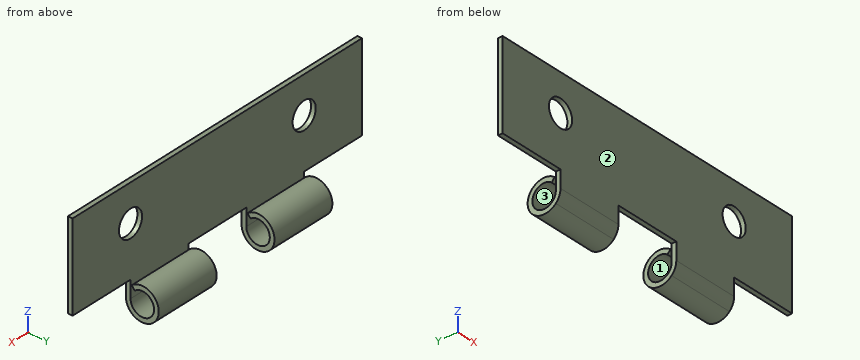
```python
from build123d import *

# Parameters (mm, degrees)
SKETCH_1_R             = 2
SM_BASE_FLANGE_1_DEPTH = 0.7
OTHER_START            = -15
OTHER_2_DEPTH          = 30
OTHER_2_2_DEPTH        = 10
OTHER_START_2          = 5
OTHER_2_3_DEPTH        = 10


# Read off the part's stored shape, not the designer's step: 褶边2
# Sheet-metal steps are written as plain solids
with BuildPart() as part:
    # Sketch 1 → 基体-法兰1 (new body)
    with BuildSketch(Plane(origin=(0, 0, 0), x_dir=(1, 0, 0), z_dir=(0, 1, 0))):
        Polygon((-25, 0), (25, 0), (25, 13), (15, 13), (15, 18), (5, 18), (5, 13), (-5, 13), (-5, 18), (-15, 18), (-15, 13), (-25, 13), align=None)
        with Locations(Location((-15, 5.5, 0), (0, 0, 270))):
            Circle(SKETCH_1_R, mode=Mode.SUBTRACT)
        with Locations(Location((15, 5.5, 0), (0, 0, 90))):
            Circle(SKETCH_1_R, mode=Mode.SUBTRACT)
    extrude(amount=-SM_BASE_FLANGE_1_DEPTH)

    # Other 2 outline → Other 2 (cut)
    with BuildSketch(Plane.YZ.offset(OTHER_START)):
        with BuildLine():
            Line((0, -18), (0, -17.264642819))
            ThreePointArc((0, -17.264642819), (-0.518259244, -16.476012959), (-0.7, -15.55))
            Line((-0.7, -15.55), (-0.7, -18))
            Line((-0.7, -18), (0, -18))
        make_face()
    extrude(amount=OTHER_2_DEPTH, mode=Mode.SUBTRACT)

    # Other 2 2 outline → Other 2 2 (add)
    with BuildSketch(Plane.YZ.offset(OTHER_START)):
        with BuildLine():
            Line((0.175170356, -13.673191114), (0.625121683, -14.209422225))
            ThreePointArc((0.625121683, -14.209422225), (3.336038627, -16.289581958), (0, -15.55))
            Line((0, -15.55), (0, -17.264642819))
            ThreePointArc((0, -17.264642819), (4.197091003, -15.669355023), (0.175170356, -13.673191114))
        make_face()
    extrude(amount=OTHER_2_2_DEPTH)

    # Other 2 3 outline → Other 2 3 (add)
    with BuildSketch(Plane.YZ.offset(OTHER_START_2)):
        with BuildLine():
            Line((0.175170356, -13.673191114), (0.625121683, -14.209422225))
            ThreePointArc((0.625121683, -14.209422225), (3.336038627, -16.289581958), (0, -15.55))
            Line((0, -15.55), (0, -17.264642819))
            ThreePointArc((0, -17.264642819), (4.197091003, -15.669355023), (0.175170356, -13.673191114))
        make_face()
    extrude(amount=OTHER_2_3_DEPTH)


solid = part.part
```
Build history of the part. All positions in model axes, mm. Face numbers are marked on the shaded views. Round coordinates to 2 decimals unless told otherwise and drop trailing zeros. Write each loop counter-clockwise with the first axis right and the second up, starting at its lowest first coordinate (ties: lowest second). Pieces come first, ordered by that corner, then holes. Notation, with made-up numbers: (59, 29) - (84, 29) arc R28 ccw to (84, 63) - close; hole circle Ø8 at (20.5, 5). An arc over 180 degrees is marked (long way). Write each question's results on one line, items separated by ' | '. Start each with the question number.
Item 1: Mould opens along Y. For the marked faces 1, 2 and 3 say: pulls with the +Y half, pulls with the -Y half, needs draft (parallel to the pull), parting line crosses it, or undercut.
Item 2: Wall check: L1, parallel to X at y = -0.6, z = -5.5; L2, parallel to Y at x = 11.75, z = -15.55; L3, parallel to Z at x = 11.5, y = 1.6. Give the ranges that are in metal, low to high. Write a range as [from, to].
Item 3: Saw through at B-B (x = -16.5). Write the cut outline in (y, z).
Item 4: Saw through at D-D (x = 11.5). Write the cut outline in (y, z), and give its area (3 significant figures).
Item 5: Drop flat-ended pins along their axis: P1, Ø0.8, axis at x = -19.5, y = 0, coming from the -Z side; P2, Ø1.5, axis at x = -11.5, y = 3, coming from the -Z side; P3, Ø1.5, axis at y = 0.5, z = -15, coming from the -X side. Give the stop position or say it passes through.
Item 6: Saw through at C-C (y = 1.25). Write the cut outline in (x, z).
Item 7: Saw through at A-A (z = -5.5). Write the cut outline in (x, y), and give its area (3 significant figures).
Results are:
1) face 1: undercut | face 2: pulls with the -Y half | face 3: undercut
2) L1: x = [-25, -17], [-13, 13], [17, 25] | L2: y = [-0.7, 0], [3.5, 4.2] | L3: z = [-18, -17.29], [-13.81, -13.1]
3) outline: (-0.7, -13) - (0, -13) - (0, -6.82) - (-0.7, -6.82) - close; (-0.7, -4.18) - (0, -4.18) - (0, 0) - (-0.7, 0) - close
4) outline: (-0.7, -15.55) arc R2.45 ccw (long way) to (0.18, -13.67) - (0.63, -14.21) arc R1.75 cw (long way) to (0, -15.55) - (0, 0) - (-0.7, 0) - close | area: 18.8 mm²
5) P1: stops at z = -13 | P2: stops at z = -17.95 | P3: stops at x = -15
6) outline: (-15, -17.95) - (-5, -17.95) - (-5, -17.23) - (-15, -17.23) - close; (-15, -13.87) - (-5, -13.87) - (-5, -13.15) - (-15, -13.15) - close; (5, -17.95) - (15, -17.95) - (15, -17.23) - (5, -17.23) - close; (5, -13.87) - (15, -13.87) - (15, -13.15) - (5, -13.15) - close
7) outline: (-25, -0.7) - (-17, -0.7) - (-17, 0) - (-25, 0) - close; (-13, -0.7) - (13, -0.7) - (13, 0) - (-13, 0) - close; (17, -0.7) - (25, -0.7) - (25, 0) - (17, 0) - close | area: 29.4 mm²
